Autodesk Inventor part; units mm, degrees
ref_plane "YZ Plane" through (0, 0, 0) normal (1, 0, 0) x (0, 1, 0)
ref_plane "XZ Plane" through (0, 0, 0) normal (0, 1, 0) x (-1, 0, 0)
ref_plane "XY Plane" through (0, 0, 0) normal (0, 0, 1) x (1, 0, 0)
sketch "Sketch1" plane through (0, 0, 0) normal (0, 1, 0) x (-1, 0, 0)
  circle A0 centre (0, 0) radius 95.25
  dimension "d0" = 190.5
extrude "Extrusion1" add sketch "Sketch1" along normal blind 184.15
shell "Shell1" thickness 3.175 removed faces 0
sketch "Sketch2" plane through (0, 184.15, 0) normal (0, 1, 0) x (1, 0, 0)
  circle A0 centre (0, 0) radius 92.075
  circle A1 centre (0, 0) radius 95.25
  dimension "d4" = 3.175
extrude "Extrusion2" cut sketch "Sketch2" against normal up to next contours A0
fillet "Fillet1" radius 3.175 1 edges at (92.075, 3.175, 0)
sketch "Sketch3" plane through (0, -30.1625, 0) normal (0, 0, 1) x (1, 0, 0)
  circle A0 centre (0, 55.5625) radius 9.525
  line L0 (120.65, 30.1625) -> (-120.65, 30.1625)
  point P0 (0, 30.1625)
  point P1 (0, 30.1625)
  point P2 (0, 30.1625)
  dimension "d12" = 19.05
  dimension "d11" = 25.4
  dimension "d16" = 0
extrude "Extrusion3" cut sketch "Sketch3" against normal through all
equation "\"d4\" = d3"
equation "\"d7\" = d3"
properties part number "HP-01" material "Aluminum 6061"
Read the model definition and answer for the solid it produces. Units are mm, in the model's axes. Round coordinates to 2 decimals unless told otherwise and drop trailing zeros. Order: outer loops, then holes, each group sorted by start corner. A loop starts at its lowest first (then second) coordinate and runs counter-clockwise, first axis right, second up.
1) Straight lines are drawn through the part: L1, parallel to Z at x = 0, y = 48.5 (3 decimals); L2, parallel to Y at x = 0, z = -93.4 (3 decimals); L3, parallel to Y at x = -58, z = -7.5 (3 decimals). For each, find the intervals that lie inside material, in ascending order.
2) The part is cut by section C-C on y = 25.4. Write down the section's boundary in (x, z) (3 decimals).
3) The mould has two halves that part along Z. Classify faces 1 (the face through (8.8, 21.75, -93.39)), 2 (the face through (75.587, 90.786, 57.958)), 3 (the face through (1, 3.175, 1)): released by +Z, released by -Z, zero draft, split by the parting line, or undercut.
4) Flat-ended cylindrical pins translate along their axes: pin 1 (8 mm diameter, centred on x = -47, y = 58.5, fed in from +Z); pin 2 (8 mm diameter, centred on x = -40.5, z = 18.5, fed in from +Y) (3 decimals); pin 3 (1 mm diameter, centred on x = -53, y = 39.5, fed in from -Z). Find the tip coordinate at first contact, or state that the pin passes through.
5) The part is cut by section A-A on y = 105. Write down the section's boundary in (x, z) (3 decimals).
Resolved:
1. L1: z = -95.25 to -92.075, 92.075 to 95.25
1. L2: y = 0 to 15.875, 34.925 to 184.15
1. L3: y = 0 to 3.175
2. outline: (-9.525, -94.773) - (-9.525, -91.581) arc R92.075 cw (long way) to (9.525, -91.581) - (9.525, -94.773) arc R95.25 ccw (long way) to start
3. face 1: zero draft
3. face 2: split by the parting line
3. face 3: undercut
4. pin 1: stops at z = 84.99
4. pin 2: stops at y = 3.175
4. pin 3: stops at z = -79.48
5. outline: circle Ø190.5 at (0, 0); hole circle Ø184.15 at (0, 0)
